from build123d import *

# Parameters (mm, degrees)
SKETCH1_R           = 40
BOSS_EXTRUDE1_DEPTH = 17.5
SHELL1_OUTLINE_R    = 30
SHELL1_DEPTH        = 7.5
CUT_EXTRUDE1_DEPTH  = 17.5


# Read off the part's stored shape, not the designer's step: Shell1
with BuildPart() as part:
    # Sketch1 → Boss-Extrude1 (new body)
    with BuildSketch(Plane.XY):
        Circle(SKETCH1_R)
        with BuildLine():
            Line((-53.841642229, 0), (-40, 0))
            ThreePointArc((-40, 0), (-39.657794455, 5.221047689), (-38.637033052, 10.352761804))
            Line((-38.637033052, 10.352761804), (-53.841642229, 14.426824554))
            Line((-53.841642229, 14.426824554), (-53.841642229, 0))
        make_face()
        with BuildLine():
            Line((-33.569714845, 42.095090962), (-24.939592074, 31.273259299))
            ThreePointArc((-24.939592074, 31.273259299), (-20.644250952, 34.260982219), (-15.995680973, 36.662490235))
            Line((-15.995680973, 36.662490235), (-22.290369216, 51.090068945))
            Line((-22.290369216, 51.090068945), (-33.569714845, 42.095090962))
        make_face()
        with BuildLine():
            Line((11.980892514, 52.491719847), (8.900837358, 38.997116487))
            ThreePointArc((8.900837358, 38.997116487), (13.914834583, 37.501698342), (18.690745131, 35.36461574))
            Line((18.690745131, 35.36461574), (26.046006457, 49.281449373))
            Line((26.046006457, 49.281449373), (11.980892514, 52.491719847))
        make_face()
        with BuildLine():
            Line((48.509643445, 23.36101305), (36.038754716, 17.355349565))
            ThreePointArc((36.038754716, 17.355349565), (37.995765867, 12.502870718), (39.302658929, 7.436464287))
            Line((39.302658929, 7.436464287), (54.769208026, 10.362893264))
            Line((54.769208026, 10.362893264), (48.509643445, 23.36101305))
        make_face()
        with BuildLine():
            ThreePointArc((36.038754716, -17.355349565), (33.46511048, -21.910873569), (30.318868926, -26.091496451))
            Line((30.318868926, -26.091496451), (42.250078864, -36.359132837))
            Line((42.250078864, -36.359132837), (48.509643445, -23.36101305))
            Line((48.509643445, -23.36101305), (36.038754716, -17.355349565))
        make_face()
        with BuildLine():
            ThreePointArc((8.900837358, -38.997116487), (3.734544338, -39.825283158), (-1.495647771, -39.972028192))
            Line((-1.495647771, -39.972028192), (-2.084221428, -55.70199032))
            Line((-2.084221428, -55.70199032), (11.980892514, -52.491719847))
            Line((11.980892514, -52.491719847), (8.900837358, -38.997116487))
        make_face()
        with BuildLine():
            ThreePointArc((-24.939592074, -31.273259299), (-28.808209861, -27.750442241), (-32.183911191, -23.752807423))
            Line((-32.183911191, -23.752807423), (-44.849060474, -33.100112979))
            Line((-44.849060474, -33.100112979), (-33.569714845, -42.095090962))
            Line((-33.569714845, -42.095090962), (-24.939592074, -31.273259299))
        make_face()
    extrude(amount=BOSS_EXTRUDE1_DEPTH)

    # Shell1 outline → Shell1 (cut)
    with BuildSketch(Plane.XY):
        Circle(SHELL1_OUTLINE_R)
    extrude(amount=SHELL1_DEPTH, mode=Mode.SUBTRACT)

    # Sketch2 → Cut-Extrude1 (cut)
    with BuildSketch(Plane(origin=(0, 0, 0), x_dir=(-1, 0, 0), z_dir=(0, 0, -1))):
        with BuildLine():
            Line((-1.223764683, -1.18), (1.223764683, -1.18))
            ThreePointArc((1.223764683, -1.18), (0, 1.7), (-1.223764683, -1.18))
        make_face()
    extrude(amount=-CUT_EXTRUDE1_DEPTH, mode=Mode.SUBTRACT)


solid = part.part
Work out the finished part from the listing and answer in its coordinate system (mm). A direction names the side the tool comes from. Give positions to 0.01 mm unless a question says otherwise; leave off trailing zeros. Loops run counter-clockwise (first coordinate to the right, second up) from the corner with the lowest first, then second, coordinate; pieces in that order, holes last. Notation, with made-up numbers: (87.5, 33.5) -> (117.5, 33.5) arc R29 ccw to (117.5, 65.5) -> close; hole circle Ø10 at (88, 49). An arc over 180 degrees is marked (long way). Use a Markdown table: item, result. Add a question column.
1) For a pull along X with two mould halves and no side action, classify faces 6 (the flat face through (42.36, -20.4, 8.63)), 7 (the cylindrical face through (-3.56, 39.84, 8.63)), 8 (the flat face through (-27.851, 46.656, 8.628)) as +X half, -X half, draft (parallel to the pull), parting line (faces both ways), or undercut.
2) The part is cut by section C-C, the plane x = 24. Determine the outline of the cut face in (y, z), plus the area to 3 significant figures.
3) Which of the six approach directions +Z, -Z, +X, -X, +Y, -Y give full straight-line access (tool end or side, diameter ignored) to faces 1 (the flat face through (42.36, 20.4, 8.63)), 2 (the cylindrical face through (-29.97, 1.32, 3.7)), 3 (the flat face through (46.93, 8.88, 8.63)), 4 (the flat face through (-47, 0, 9)), 5 (the flat face through (0, -1.18, 12))?
4) Each of these flat-tipped pins is pushed along its axis until it touches: P1, Ø5.5, axis at x = 0, y = 0, coming from the -Z side; P2, Ø5, axis at x = 17.5, z = 15, coming from the +Y side; P3, Ø2.5, axis at x = 0.5, z = 10.5, coming from the +Y side. Where does it stop, or does it pass through?
5) The part is cut by section B-B, the plane y = 22. Determine the outline of the cut face in (x, z).
6) Consider line 1 along Z through (x, y) = (24.5, 3.5); line 2 along X through (y, z) = (-40, 14); line 3 along Y through (x, z) = (47, 13.25). Determine where each line is inside the solid, lowest interval first.
Reported:
| question | item | result |
|---|---|---|
| 1 | face 6 | +X half |
| 1 | face 7 | undercut |
| 1 | face 8 | -X half |
| 2 | outline | (-32, 0) -> (-18, 0) -> (-18, 7.5) -> (18, 7.5) -> (18, 0) -> (32, 0) -> (32, 17.5) -> (-32, 17.5) -> close; (45.41, 0) -> (49.75, 0) -> (49.75, 17.5) -> (45.41, 17.5) -> close |
| 2 | area | 926 mm^2 |
| 3 | face 1 | +Z, -Z, +Y |
| 3 | face 2 | -Z |
| 3 | face 3 | +Z, -Z, +X |
| 3 | face 4 | +Z, -Z, -X |
| 3 | face 5 | +Z, -Z |
| 4 | P1 | stops at z = 7.5 |
| 4 | P2 | stops at y = 51.8 |
| 4 | P3 | stops at y = 40 |
| 5 | outline | (-33.41, 0) -> (-20.4, 0) -> (-20.4, 7.5) -> (20.4, 7.5) -> (20.4, 0) -> (33.41, 0) -> (33.41, 17.5) -> (-33.41, 17.5) -> close; (45.68, 0) -> (49.17, 0) -> (49.17, 17.5) -> (45.68, 17.5) -> close |
| 6 | line 1 | z = 7.5 to 17.5 |
| 6 | line 2 | x = -36.2 to -31.9, -1.5 to 9.13 |
| 6 | line 3 | y = -26.5 to -22.63, 8.89 to 22.63 |
